```python
from build123d import *

# Parameters (mm, degrees)
SKETCH1_R                = 14.1
BOSS_EXTRUDE1_DEPTH      = 9.3
SKETCH2_W                = 7.1
SKETCH2_H                = 2.8
BOSS_EXTRUDE2_DEPTH      = 0.35
BOSS_EXTRUDE2_DEPTH_BACK = 9.65
SKETCH3_R                = 9.85
CHAMFER1_SIZE            = 0.35
SKETCH4_R                = 7
BOSS_EXTRUDE3_DEPTH      = 6
CUT_EXTRUDE1_REACH       = 27.566
SKETCH5_R                = 3
CHAMFER2_SIZE            = 0.2


with BuildPart() as part:
    # Sketch1 → Boss-Extrude1 (new body)
    with BuildSketch(Plane.XY):
        Circle(SKETCH1_R)
    extrude(amount=BOSS_EXTRUDE1_DEPTH)

    # Sketch2 → Cut-Revolve1 (revolve, cut)
    with BuildSketch(Plane(origin=(0, 0, 0), x_dir=(0, 0, -1), z_dir=(1, 0, 0)), mode=Mode.PRIVATE) as cut_revolve1_sk:
        with Locations((-4.65, 12.7)):
            Rectangle(SKETCH2_W, SKETCH2_H)
    revolve(cut_revolve1_sk.sketch.rotate(Axis((0, 0, -195813.923931263), (0, 0, -1)), 270), axis=Axis((0, 0, -195813.923931263), (0, 0, -1)), mode=Mode.SUBTRACT)

    # Sketch3 → Boss-Extrude2 (add, two sides: drawn at the far end of the back side and taken through both)
    with BuildSketch(Plane.XY.offset(9.3).offset(-BOSS_EXTRUDE2_DEPTH_BACK)):
        Circle(SKETCH3_R)
    extrude(amount=BOSS_EXTRUDE2_DEPTH + BOSS_EXTRUDE2_DEPTH_BACK)

    # Chamfer1
    chamfer1_edges = [part.edges().sort_by_distance(p)[0] for p in [
        (-9.85, 0, -0.35),
        (-9.85, 0, 9.65),
    ]]
    chamfer(chamfer1_edges, length=CHAMFER1_SIZE - 0.0001)  # a hair under: the kernel refuses the full size

    # Sketch4 → Boss-Extrude3 (add)
    with BuildSketch(Plane(origin=(0, 0, -0.35), x_dir=(-1, 0, 0), z_dir=(0, 0, -1))):
        with Locations(Location((0, 0, 0), (0, 0, 180))):
            Circle(SKETCH4_R)
    extrude(amount=BOSS_EXTRUDE3_DEPTH)

    # Sketch5 → Cut-Extrude1 (cut, up to next)
    with BuildSketch(Plane(origin=(0, 0, -6.35), x_dir=(-1, 0, 0), z_dir=(0, 0, -1)), mode=Mode.PRIVATE) as cut_extrude1_sk1:
        Circle(SKETCH5_R)
    cut_extrude1_tool1 = extrude(cut_extrude1_sk1.sketch, amount=-CUT_EXTRUDE1_REACH, mode=Mode.PRIVATE) & part.part
    add(cut_extrude1_tool1.solids().sort_by_distance((0, 0, -6.35))[0], mode=Mode.SUBTRACT)

    # Chamfer2
    chamfer2_edges = [part.edges().sort_by_distance(p)[0] for p in [
        (-14.1, 0, 0),
        (-7, 0, -6.35),
        (3, 0, 9.65),
        (3, 0, -6.35),
        (-14.1, 0, 9.3),
        (-14.1, 0, 1.1),
        (-14.1, 0, 8.2),
    ]]
    chamfer(chamfer2_edges, length=CHAMFER2_SIZE)


solid = part.part
```
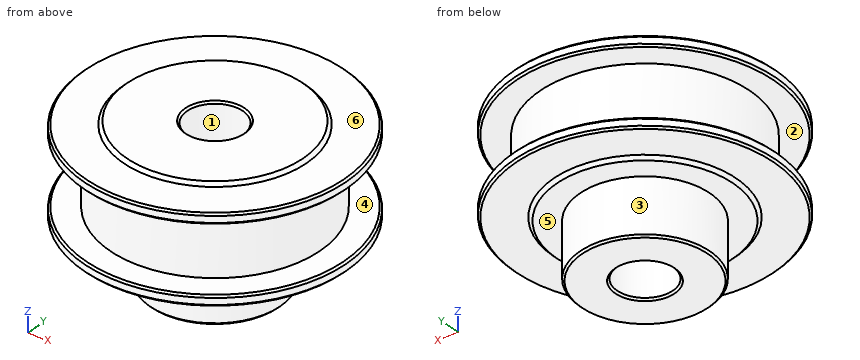
Check sheet for the modelled part. Datum: model origin and axes. Units: mm. Face numbers are marked on the shaded views. A direction names the side the tool comes from. Round coordinates to 2 decimals unless told otherwise and drop trailing zeros. Order: outer loops, then holes, each group sorted by start corner. A loop starts at its lowest first (then second) coordinate and runs counter-clockwise, first axis right, second up. Notation, with made-up numbers: (56, 60.5) - (63, 60.5) arc R27 ccw to (63, 81.5) - close; hole circle Ø11 at (-12, 17.25). An arc over 180 degrees is marked (long way). Answer as CSV lines item,"result". Start each with the question number.
1) Scan lines: probe 1 along Y at (x, z) = (0, 1.75); probe 2 along Z at (x, y) = (6.25, -8.75); probe 3 along Y at (x, z) = (0, -2.5). Record each from-to range of solid material in increasing order.
2) Depth check by flat-ended pin: pin 1 (4 mm diameter, centred on x = 4.5, z = 5.5, fed in from +Y); pin 2 (10 mm diameter, centred on x = -0.5, y = 10.5, fed in from -Z); pin 3 (1 mm diameter, centred on y = -4, z = 3, fed in from -X); pin 4 (1.5 mm diameter, centred on x = -7, y = 7, fed in from -Z). Enter the tip coordinate at first touch or a pass-through.
3) Section check A-A (z = 2.75). Record the cut outline in (x, y), then the cut area to 3 significant figures.
4) Draft check along Y on the marked faces 1, 2 and 3. Enter one of: +Y half, -Y half, draft (parallel to the pull), parting line (faces both ways), or undercut.
5) Section check B-B (z = -5). Record the cut outline in (x, y).
6) Tool access check on the marked faces 4, 5 and 6. Record the directions out of +Z, -Z, +X, -X, +Y, -Y that give a thin tool (end or side, any length) a straight path to the whole face; none if there is none.
Determined:
1,probe 1,"-11.3 to -3, 3 to 11.3"
1,probe 2,"0 to 9.3"
1,probe 3,"-7 to -3, 3 to 7"
2,pin 1,"y = 11.02"
2,pin 2,"z = -6.35"
2,pin 3,"x = -10.74"
2,pin 4,"z = -0.35"
3,outline,"circle Ø22.6 at (0, 0); hole circle Ø6 at (0, 0)"
3,area,"373 mm^2"
4,face 1,"undercut"
4,face 2,"draft"
4,face 3,"parting line"
5,outline,"circle Ø14 at (0, 0); hole circle Ø6 at (0, 0)"
6,face 4,"none"
6,face 5,"-Z"
6,face 6,"+Z"
